from build123d import *

# Parameters (mm, degrees)
SKETCH1_W           = 30
SKETCH1_H           = 110
SKETCH1_R           = 10
BOSS_EXTRUDE1_DEPTH = 15
CHAMFER1_SIZE       = 1


with BuildPart() as part:
    # Sketch1 → Boss-Extrude1 (new body)
    with BuildSketch(Plane.XY):
        Rectangle(SKETCH1_W, SKETCH1_H)
        with Locations((0, 43)):
            Circle(SKETCH1_R, mode=Mode.SUBTRACT)
        with Locations((0, -43)):
            Circle(SKETCH1_R, mode=Mode.SUBTRACT)
    extrude(amount=BOSS_EXTRUDE1_DEPTH)

    # Chamfer1
    chamfer1_edges = [part.edges().sort_by_distance(p)[0] for p in [
        (-15, 0, 15),
        (-10, 43, 0),
        (-10, 43, 15),
        (0, -55, 15),
        (-10, -43, 0),
        (-10, -43, 15),
        (15, 0, 15),
        (0, -55, 0),
        (-15, 0, 0),
        (0, 55, 0),
        (15, 0, 0),
        (0, 55, 15),
        (15, -55, 7.5),
        (-15, -55, 7.5),
        (-15, 55, 7.5),
        (15, 55, 7.5),
    ]]
    chamfer(chamfer1_edges, length=CHAMFER1_SIZE - 0.0001)  # a hair under: the kernel refuses the full size


solid = part.part
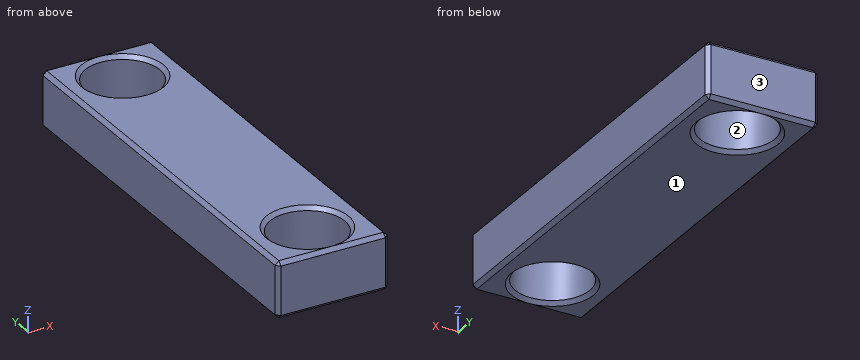
Geometry: final body of the model. Coordinates: model frame, mm. Face numbers are marked on the shaded views. Give positions to 0.01 mm unless a question says otherwise; leave off trailing zeros. Write each loop counter-clockwise with the first axis right and the second up, starting at its lowest first coordinate (ties: lowest second). Pieces come first, ordered by that corner, then holes. Notation, with made-up numbers: (48.5, 6.25) -> (69.5, 6.25) arc R30 ccw to (69.5, 35.25) -> close; hole circle Ø3 at (63, 61.5). An arc over 180 degrees is marked (long way). Answer as a JSON object with one key per item and string values.
1. Cut plane C-C on x = 0. Count the separate pieces of the cut face and the enclosed holes in it, and give its area (3 significant figures).
Ans:
{"separate pieces": "3", "enclosed holes": "0", "area": "1,040 mm^2"}
2. Cut plane A-A on y = -43. Output: boundary loops of the cut face in (x, z), and give its area (3 significant figures).
Ans:
{"outline": "(-15, 1) -> (-14, 0) -> (-11, 0) -> (-10, 1) -> (-10, 14) -> (-11, 15) -> (-14, 15) -> (-15, 14) -> close; (10, 1) -> (11, 0) -> (14, 0) -> (15, 1) -> (15, 14) -> (14, 15) -> (11, 15) -> (10, 14) -> close", "area": "146 mm^2"}
3. Ray query, probe 1 along Y at (x, z) = (0, 4.75); probe 2 along Y at (x, z) = (1, 8); probe 3 along X at (y, z) = (42.5, 8.75). Return the intervals inside material, ascending. Write a range as from..to.
Ans:
{"probe 1": "y = -55..-53, -33..33, 53..55", "probe 2": "y = -55..-52.95, -33.05..33.05, 52.95..55", "probe 3": "x = -15..-9.99, 9.99..15"}
4. Mould query, pull axis Y, two halves, no side actions, for the marked faces 1, 2 and 3. Classes: pulls with the +Y half, pulls with the -Y half, needs draft (parallel to the pull), parting line crosses it, or undercut.
Ans:
{"face 1": "needs draft", "face 2": "undercut", "face 3": "pulls with the +Y half"}
5. Contact query for a flat-ended pin moving along its axis: pin 1 (18 mm diameter, centred on x = 0, y = 43, fed in from +Z). Output: stop coordinate, or through.
Ans:
{"pin 1": "passes through"}
6. Cut plane B-B on z = 11.75. Output: boundary loops of the cut face in (x, y), and give its area (3 significant figures).
Ans:
{"outline": "(-15, -54) -> (-14, -55) -> (14, -55) -> (15, -54) -> (15, 54) -> (14, 55) -> (-14, 55) -> (-15, 54) -> close; hole circle Ø20 at (0, -43); hole circle Ø20 at (0, 43)", "area": "2,670 mm^2"}
